Verification items for this drawing (mm, ordinates from the low corner). A direction names the side the tool comes from. Round coordinates to 2 decimals unless told otherwise and drop trailing zeros. Loops run counter-clockwise (first coordinate to the right, second up) from the corner with the lowest first, then second, coordinate; pieces in that order, holes last. Notation, with made-up numbers: (79.5, -3.5) - (118.5, -3.5) arc R29 cw to (118.5, 34.5) - close; hole circle Ø2 at (16, 28.25). An arc over 180 degrees is marked (long way). Answer in a Markdown table with one row per item. Add a question column.
(1) Thickness scan on line 1 along Y through (x, z) = (8.5, 2.35); line 2 along Y through (x, z) = (15, 9); line 3 along Z through (x, y) = (1, 33). Record the ranges inside material, lowest first.
(2) Cross-section at B-B on x = 8.5. Count the separate pieces of the cut face and the enclosed holes in it, then the cut area to 3 significant figures.
(3) Access from +Z, -Z, +X, -X, +Y, -Y to the whole of each face (thin tool, end or side, straight path). Record for the marked faces 4, 5, 6, 7 and 8.
(4) Gauge pin test, flat ends, axial feed: pin 1 (0.9 mm diameter, centred on x = 7.5, y = 9.5, fed in from +Z); pin 2 (3 mm diameter, centred on x = 13, y = 35, fed in from +Z); pin 3 (10 mm diameter, centred on x = 6, z = 27, fed in from -Y). Record the tip position at first contact, or that the pin passes through.
(5) Cross-section at A-A on z = 8.5. Enter the section's corners in (x, y).
(6) Cross-section at C-C on y = 36. Enter the section's corners in (x, z), then the cut area to 3 significant figures.
(7) Cross-section at D-D on z = 17. Enter the section's corners in (x, y).
(8) Mould release check, pull along Y, two halves, no side actions. Record for the marked faces 1, 2 and 3: +Y half, -Y half, draft (parallel to the pull), parting line (faces both ways), or undercut.
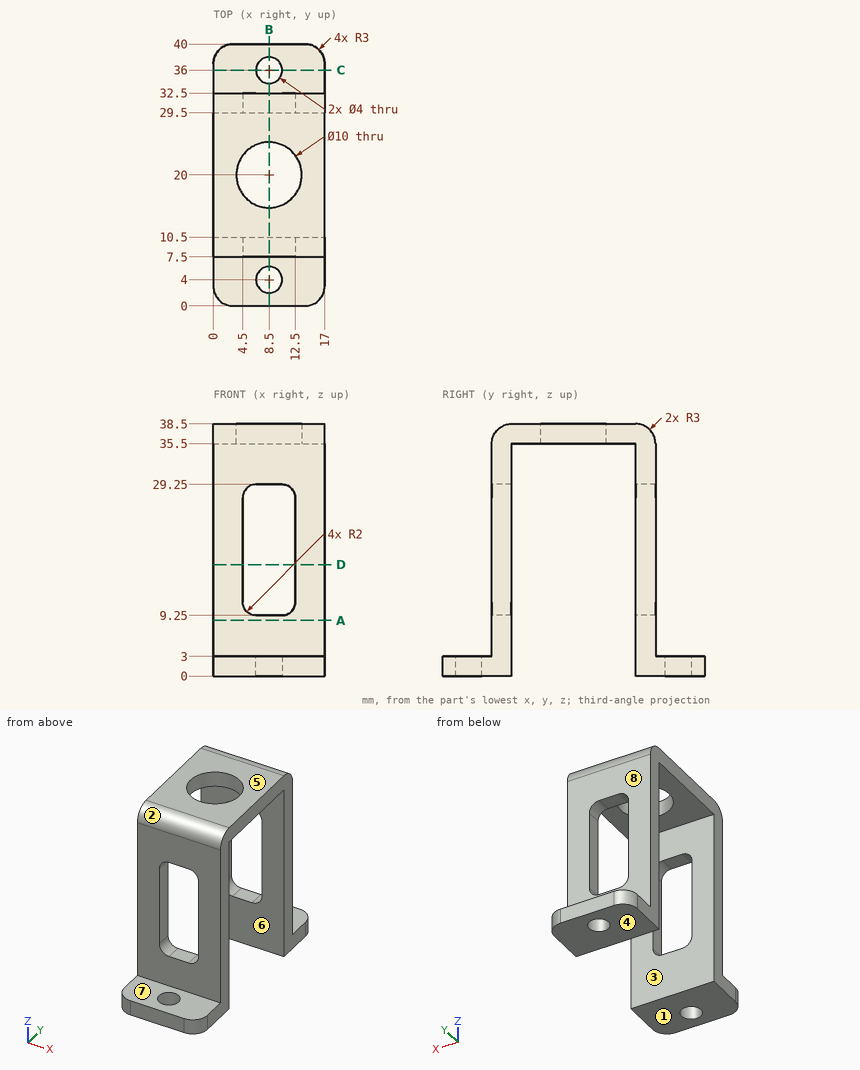
Answers:
| question | item | result |
|---|---|---|
| 1 | line 1 | y = 0 to 2, 6 to 10.5, 29.5 to 34, 38 to 40 |
| 1 | line 2 | y = 7.5 to 10.5, 29.5 to 32.5 |
| 1 | line 3 | z = 0 to 3 |
| 2 | separate pieces | 6 |
| 2 | enclosed holes | 0 |
| 2 | area | 155 mm^2 |
| 3 | face 4 | -Z, +X, -X, +Y, -Y |
| 3 | face 5 | +Z, +X, -X, +Y, -Y |
| 3 | face 6 | -Z, +X, -X |
| 3 | face 7 | +Z, +X, -X, -Y |
| 3 | face 8 | +Z, +X, -X, +Y |
| 4 | pin 1 | stops at z = 38.45 |
| 4 | pin 2 | stops at z = 3 |
| 4 | pin 3 | stops at y = 7.5 |
| 5 | outline | (0, 7.5) - (17, 7.5) - (17, 10.5) - (0, 10.5) - close; (0, 29.5) - (17, 29.5) - (17, 32.5) - (0, 32.5) - close |
| 6 | outline | (0, 0) - (6.5, 0) - (6.5, 3) - (0, 3) - close; (10.5, 0) - (17, 0) - (17, 3) - (10.5, 3) - close |
| 6 | area | 39.0 mm^2 |
| 7 | outline | (0, 7.5) - (4.5, 7.5) - (4.5, 10.5) - (0, 10.5) - close; (0, 29.5) - (4.5, 29.5) - (4.5, 32.5) - (0, 32.5) - close; (12.5, 7.5) - (17, 7.5) - (17, 10.5) - (12.5, 10.5) - close; (12.5, 29.5) - (17, 29.5) - (17, 32.5) - (12.5, 32.5) - close |
| 8 | face 1 | draft |
| 8 | face 2 | -Y half |
| 8 | face 3 | undercut |
